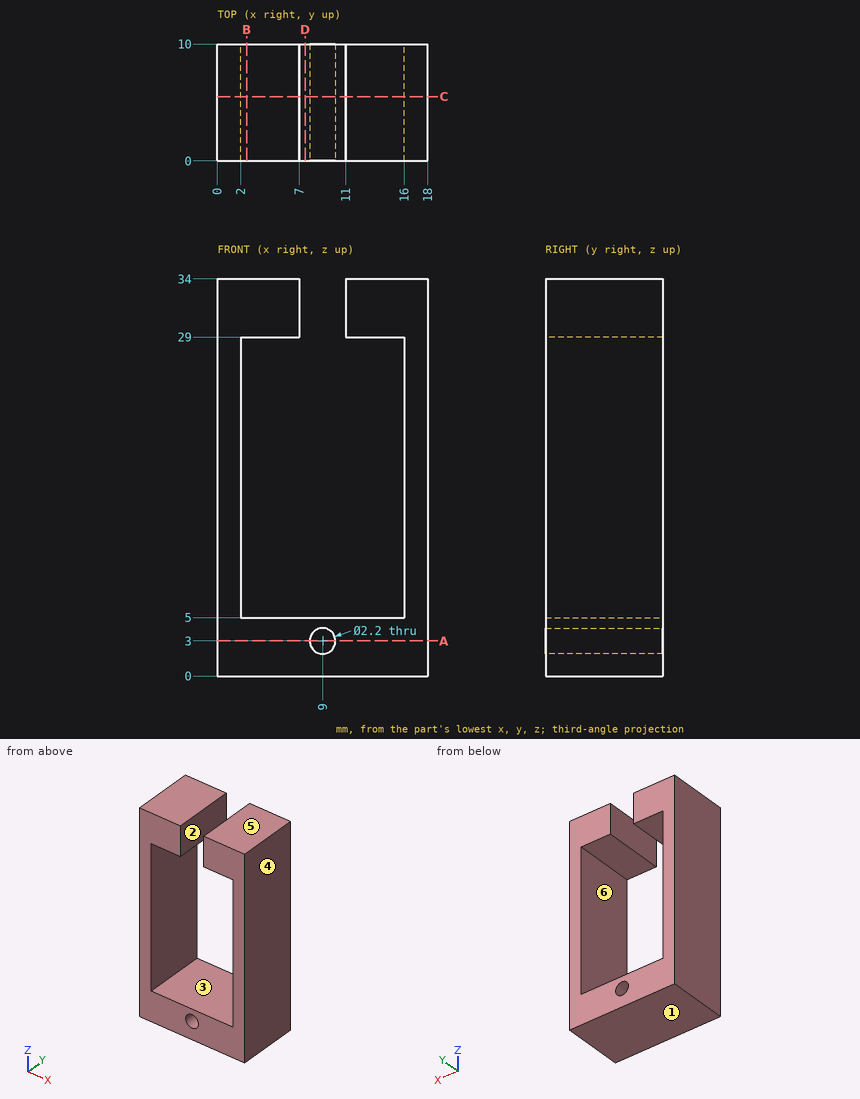
Geometry check sheet. Reference: drawing and pictorial views, mm from the part's lowest x, y, z. A direction names the side the tool comes from. Round coordinates to 2 decimals unless told otherwise and drop trailing zeros. Order: outer loops, then holes, each group sorted by start corner. A loop starts at its lowest first (then second) coordinate and runs counter-clockwise, first axis right, second up. Notation, with made-up numbers: M 74.25,80 L 87.25,80 A17 cw 87.25,98 Z; hole C -8,62 d6. An arc over 180 degrees is marked long. One line per item, written item: value. Start each with the question number.
1. Release check for a two-part mould opening along X. For the marked faces 4, 5 and 6 record: released by +X, released by -X, zero draft, split by the parting line, or undercut.
2. Section check D-D on x = 7.5. Enter the section's corners in (y, z).
3. Scan lines: line 1 along X through (y, z) = (5, 3); line 2 along X through (y, z) = (5.5, 20); line 3 along Z through (x, y) = (4.75, 3.75). Record each from-to range of solid material in increasing order.
4. Section check A-A on z = 3. Enter the section's corners in (x, y), and give its area (3 significant figures).
5. Access from +Z, -Z, +X, -X, +Y, -Y to the whole of each face (thin tool, end or side, straight path). Record for the marked faces 1, 2 and 3.
6. Section check C-C on y = 5.5. Enter the section's corners in (x, z).
7. Section check B-B on x = 2.5. Enter the section's corners in (y, z).
8. Gauge pin test, flat end, axial feed: P1, Ø10, axis at x = 12.5, z = 30.5, coming from the -Y side. Record the tip position at first contact, or that the pin passes through.
Results found:
1. face 4: released by +X
1. face 5: zero draft
1. face 6: undercut
2. outline: M 0,0 L 10,0 L 10,5 L 0,5 Z
3. line 1: 0 to 7.9, 10.1 to 18
3. line 2: 0 to 2, 16 to 18
3. line 3: 0 to 5, 29 to 34
4. outline: M 0,0 L 7.9,0 L 7.9,10 L 0,10 Z; M 10.1,0 L 18,0 L 18,10 L 10.1,10 Z
4. area: 158 mm^2
5. face 1: -Z, +X, -X, +Y, -Y
5. face 2: +Z, +Y, -Y
5. face 3: +Y, -Y
6. outline: M 0,0 L 18,0 L 18,34 L 11,34 L 11,29 L 16,29 L 16,5 L 2,5 L 2,29 L 7,29 L 7,34 L 0,34 Z; hole C 9,3 d2.2
7. outline: M 0,0 L 10,0 L 10,5 L 0,5 Z; M 0,29 L 10,29 L 10,34 L 0,34 Z
8. P1: y = 0
